Geometry check sheet. Reference: the model listing, model coordinates, mm. A direction names the side the tool comes from. Coordinates: 2 decimals unless noted, no trailing zeros. Write each loop counter-clockwise with the first axis right and the second up, starting at its lowest first coordinate (ties: lowest second). Pieces come first, ordered by that corner, then holes. Notation, with made-up numbers: (40, 67.5) - (98, 67.5) arc R22 ccw to (98, 77.5) - close; hole circle Ø1 at (43, 22.25). An arc over 180 degrees is marked (long way). Answer as a JSON object with one key per item and string values. Group by question number.
from build123d import *

# Parameters (mm, degrees)
SKETCH_1_W      = 30
SKETCH_1_H      = 30
EXTRUDE_1_DEPTH = 15
SKETCH_5_R      = 1.5
EXTRUDE_2_DEPTH = 2
FILLET_1_R      = 2


with BuildPart() as part:
    # Эскиз1 → Бобышка-Вытянуть1 (new body, symmetric)
    with BuildSketch(Plane(origin=(0, 0, 0), x_dir=(1, 0, 0), z_dir=(0, 1, 0))):
        Rectangle(SKETCH_1_W, SKETCH_1_H)
    extrude(amount=EXTRUDE_1_DEPTH, both=True)

    # Эскиз4 → Вырез-Повернуть1 (revolve, cut)
    with BuildSketch(Plane.XY):
        Polygon((-4.5, -15), (-4.5, -14), (-8.75, -9.75), (-8.75, 14), (-9.75, 15), (0, 15), (0, -15), align=None)
    cut_revolve_1 = revolve(axis=Axis((0, 15, 0), (0, -1, 0)), mode=Mode.SUBTRACT)

    # Эскиз5 → Бобышка-Вытянуть2 (add)
    with BuildSketch(Plane.XZ.offset(15)):
        with Locations(Location((-10, 7.5, 0), (0, 0, 270))):  # turned: the seam where the file's is
            Circle(SKETCH_5_R)
        with Locations(Location((-10, -7.5, 0), (0, 0, 270))):  # turned: the seam where the file's is
            Circle(SKETCH_5_R)
        with Locations(Location((10, -7.5, 0), (0, 0, 270))):  # turned: the seam where the file's is
            Circle(SKETCH_5_R)
        with Locations(Location((10, 7.5, 0), (0, 0, 270))):  # turned: the seam where the file's is
            Circle(SKETCH_5_R)
    extrude_2 = extrude(amount=EXTRUDE_2_DEPTH)

    # Зеркальное отражение1: Вырез-Повернуть1, Бобышка-Вытянуть2 across plane
    add(cut_revolve_1.mirror(Plane(origin=(0, 0, 0), x_dir=(0, 0, 1), z_dir=(0.707106781, 0.707106781, 0))), mode=Mode.SUBTRACT)
    add(extrude_2.mirror(Plane(origin=(0, 0, 0), x_dir=(0, 0, 1), z_dir=(0.707106781, 0.707106781, 0))))

    # Скругление1
    fillet_1_edges = [part.edges().sort_by_distance(p)[0] for p in [
        (-15, 15, 0),
        (0, 15, 15),
        (15, 15, 0),
        (-15, -15, 0),
        (0, -15, -15),
        (-15, 0, 15),
        (-15, 0, -15),
        (15, 0, -15),
        (0, 15, -15),
    ]]
    fillet(fillet_1_edges, radius=FILLET_1_R)

    # Зеркальное отражение2: Вырез-Повернуть1, Бобышка-Вытянуть2 across plane
    add(cut_revolve_1.mirror(Plane(origin=(0, 0, 0), x_dir=(0, -0.707106781, 0.707106781), z_dir=(0, 0.707106781, 0.707106781))), mode=Mode.SUBTRACT)
    add(extrude_2.mirror(Plane(origin=(0, 0, 0), x_dir=(0, -0.707106781, 0.707106781), z_dir=(0, 0.707106781, 0.707106781))))


solid = part.part
(1) Section check A-A (y = -12). Record the cut outline in (x, z).
(2) Section check D-D (x = 15.5). Record the cut outline in (y, z).
(3) Section check C-C (z = 12.5). Record the cut outline in (x, y).
(4) Set-up check for faces 4 (the face through (9.1, -8.7, 16)), 5 (the face through (-11.016, -1.139, -8.676)), 6 (the face through (1.139, 11.016, -8.676)), 7 (the face through (6.45, 5.91, 8.74)): record each of +Z, -Z, +X, -X, +Y, -Y from which the full face is reachable in a straight line by a thin tool's end or side.
(5) Draft check along X on faces 1 (the face through (16, 10.9, 8.7)), 2 (the face through (6.45, -8.74, -5.91)), 3 (the face through (-14.43, -0.18, -14.4)). Enter one of: +X half, -X half, draft (parallel to the pull), parting line (faces both ways), or undercut.
(6) Material ranges on L1, parallel to Z at x = -7.5, y = -9; L2, parallel to Z at x = -11, y = 0; L3, parallel to Y at x = 15.5, z = 7.5, recorded low to high. Write a range as [from, to].
(7) Section check B-B (z = 0). Count the separate pieces of the cut face and the enclosed holes in it, and give its area (3 significant figures).
(8) Gauge pin test, flat ends, axial feed: pin 1 (3 mm diameter, centred on x = 5.5, z = -1.5, fed in from -Y); pin 2 (8 mm diameter, centred on y = 0, z = 0, fed in from -X); pin 3 (3 mm diameter, centred on x = 2, y = -7.5, fed in from +Z); pin 4 (16 mm diameter, centred on y = 0, z = 0, fed in from +X). Record the tip position at first contact, or that the pin passes through.
Conclusion:
{
 "1": {"outline": "(-15, -13) arc R2 ccw to (-13, -15) - (13, -15) arc R2 ccw to (15, -13) - (15, 15) - (-13, 15) arc R2 ccw to (-15, 13) - close; hole circle Ø13 at (0, 0)"},
 "2": {"outline": "circle Ø3 at (-10, -7.5); circle Ø3 at (-10, 7.5); circle Ø3 at (10, -7.5); circle Ø3 at (10, 7.5)"},
 "3": {"outline": "(-15, -13) arc R2 ccw to (-13, -15) - (15, -15) - (15, 13) arc R2 ccw to (13, 15) - (-13, 15) arc R2 ccw to (-15, 13) - close; hole circle Ø12 at (0, 0)"},
 "4": {"face 4": "+Z", "face 5": "-X", "face 6": "+Y", "face 7": "-Z"},
 "5": {"face 1": "draft", "face 2": "undercut", "face 3": "-X half"},
 "6": {"L1": "z = [-15, -4.51], [4.51, 15]", "L2": "z = [-15, -8.75], [8.75, 15]", "L3": "y = [-11.5, -8.5], [8.5, 11.5]"},
 "7": {"separate pieces": "4", "enclosed holes": "0", "area": "205 mm^2"},
 "8": {"pin 1": "stops at y = -15", "pin 2": "passes through", "pin 3": "stops at z = 15", "pin 4": "stops at x = 15"}
}
